Verification items for the finished model (mm, model axes). Coordinates: 2 decimals unless noted, no trailing zeros. Write each loop counter-clockwise with the first axis right and the second up, starting at its lowest first coordinate (ties: lowest second). Pieces come first, ordered by that corner, then holes. Notation, with made-up numbers: (-5, 44.5) -> (43, 44.5) arc R23 ccw to (43, 62.5) -> close; hole circle Ø5 at (69.5, 23). An arc over 180 degrees is marked (long way). Write item = value, one per line. Start each with the question number.
(1) Mould release check, pull along Z, two halves, no side actions. Record for faces 1 (the face through (-44, -154, 26)), 2 (the face through (15.02, -2.15, 47.69)), 3 (the face through (2.64, -2.15, -59.94)): released by +Z, released by -Z, zero draft, split by the parting line, or undercut.
(2) Gauge pin test, flat ends, axial feed: pin 1 Ø3 at (x, z) = (-55, 0) entering from +Y; pin 2 Ø4 at (y, z) = (-120.5, -41) entering from +X; pin 3 Ø3 at (x, y) = (-23, -37) entering from +Z. Record the tip position at first contact, or that the pin passes through.
(3) Section check A-A (y = 126.5). Record the cut outline in (x, z), plus the area to 3 significant figures.
(4) Material ranges on probe 1 along X at (y, z) = (145, 0); probe 2 along X at (y, z) = (125.5, 2); probe 3 along X at (y, z) = (122, -8.5), recorded low to high. Write a range as [from, to].
```python
from build123d import *

# Parameters (mm, degrees)
BOSS_EXTRUDE1_DEPTH              = 154
BOSS_EXTRUDE1_DEPTH_BACK         = 154
SKETCH1_R                        = 60
SKETCH1_R_2                      = 50
TAP_DRILL_FOR_M6_TAP1_AT_2_COUNT = 2
TAP_DRILL_FOR_M6_TAP1_AT_2_PITCH = 42.09517756
TAP_DRILL_FOR_M6_TAP1_AT_3_COUNT = 2
TAP_DRILL_FOR_M6_TAP1_AT_3_PITCH = 77.781745931
TAP_DRILL_FOR_M6_TAP1_AT_4_COUNT = 2
TAP_DRILL_FOR_M6_TAP1_AT_4_PITCH = 101.626748576
TAP_DRILL_FOR_M6_TAP1_AT_5_COUNT = 2
TAP_DRILL_FOR_M6_TAP1_AT_5_PITCH = 110
TAP_DRILL_FOR_M6_TAP1_AT_6_COUNT = 2
TAP_DRILL_FOR_M6_TAP1_AT_6_PITCH = 101.626748576
TAP_DRILL_FOR_M6_TAP1_AT_7_COUNT = 2
TAP_DRILL_FOR_M6_TAP1_AT_7_PITCH = 77.781745931
TAP_DRILL_FOR_M6_TAP1_AT_8_COUNT = 2
TAP_DRILL_FOR_M6_TAP1_AT_8_PITCH = 42.09517756
CHAMFER1_SIZE                    = 0.6


with BuildPart() as part:
    # Sketch1 → Boss-Extrude1 (new, two sides: drawn at the far end of the back side and taken through both)
    with BuildSketch(Plane(origin=(0, 0, 0), x_dir=(1, 0, 0), z_dir=(0, 1, 0)).offset(-BOSS_EXTRUDE1_DEPTH_BACK)):
        with Locations(Location((0, 0, 0), (0, 0, 270))):
            Circle(SKETCH1_R)
        with Locations(Location((0, 0, 0), (0, 0, 270))):
            Circle(SKETCH1_R_2, mode=Mode.SUBTRACT)
    extrude(amount=BOSS_EXTRUDE1_DEPTH + BOSS_EXTRUDE1_DEPTH_BACK)

    # Sketch3 → Tap Drill for M6 Tap1 (revolve, cut)
    with BuildSketch(Plane(origin=(-38.890872965, 154, -38.890872965), x_dir=(0, 0, 1), z_dir=(1, 0, 0))):
        Polygon((0, 0), (0, 16.502151548), (2.5, 15), (2.5, 0), align=None)
    tap_drill_for_m6_tap1 = revolve(axis=Axis((-38.890872965, 160.35, -38.890872965), (0, -1, 0)), mode=Mode.SUBTRACT)

    # Tap Drill for M6 Tap1 at 2: Tap Drill for M6 Tap1 ×2
    with Locations(*[Vector(0.92387953251135, 0, -0.3826834323649371) * (i * TAP_DRILL_FOR_M6_TAP1_AT_2_PITCH) for i in range(1, TAP_DRILL_FOR_M6_TAP1_AT_2_COUNT)]):
        add(tap_drill_for_m6_tap1, mode=Mode.SUBTRACT)

    # Tap Drill for M6 Tap1 at 3: Tap Drill for M6 Tap1 ×2
    with Locations(*[(i * TAP_DRILL_FOR_M6_TAP1_AT_3_PITCH, 0, 0) for i in range(1, TAP_DRILL_FOR_M6_TAP1_AT_3_COUNT)]):
        add(tap_drill_for_m6_tap1, mode=Mode.SUBTRACT)

    # Tap Drill for M6 Tap1 at 4: Tap Drill for M6 Tap1 ×2
    with Locations(*[Vector(0.9238795325112054, 0, 0.3826834323652862) * (i * TAP_DRILL_FOR_M6_TAP1_AT_4_PITCH) for i in range(1, TAP_DRILL_FOR_M6_TAP1_AT_4_COUNT)]):
        add(tap_drill_for_m6_tap1, mode=Mode.SUBTRACT)

    # Tap Drill for M6 Tap1 at 5: Tap Drill for M6 Tap1 ×2
    with Locations(*[Vector(0.7071067811863805, 0, 0.7071067811867146) * (i * TAP_DRILL_FOR_M6_TAP1_AT_5_PITCH) for i in range(1, TAP_DRILL_FOR_M6_TAP1_AT_5_COUNT)]):
        add(tap_drill_for_m6_tap1, mode=Mode.SUBTRACT)

    # Tap Drill for M6 Tap1 at 6: Tap Drill for M6 Tap1 ×2
    with Locations(*[Vector(0.38268343236484964, 0, 0.9238795325113862) * (i * TAP_DRILL_FOR_M6_TAP1_AT_6_PITCH) for i in range(1, TAP_DRILL_FOR_M6_TAP1_AT_6_COUNT)]):
        add(tap_drill_for_m6_tap1, mode=Mode.SUBTRACT)

    # Tap Drill for M6 Tap1 at 7: Tap Drill for M6 Tap1 ×2
    with Locations(*[(0, 0, i * TAP_DRILL_FOR_M6_TAP1_AT_7_PITCH) for i in range(1, TAP_DRILL_FOR_M6_TAP1_AT_7_COUNT)]):
        add(tap_drill_for_m6_tap1, mode=Mode.SUBTRACT)

    # Tap Drill for M6 Tap1 at 8: Tap Drill for M6 Tap1 ×2
    with Locations(*[Vector(-0.38268343236537383, 0, 0.9238795325111692) * (i * TAP_DRILL_FOR_M6_TAP1_AT_8_PITCH) for i in range(1, TAP_DRILL_FOR_M6_TAP1_AT_8_COUNT)]):
        add(tap_drill_for_m6_tap1, mode=Mode.SUBTRACT)

    # Mirror1: Tap Drill for M6 Tap1 across plane
    add(tap_drill_for_m6_tap1.mirror(Plane.ZX), mode=Mode.SUBTRACT)

    # Mirror1 copy 1 sketch → Mirror1 copy 1 (revolve, cut)
    with BuildSketch(Plane(origin=(0, -154, -55), x_dir=(0, 0, 1), z_dir=(1, 0, 0))):
        Polygon((0, 0), (0, -16.502151548), (2.5, -15), (2.5, 0), align=None)
    revolve(axis=Axis((0, -160.35, -55), (0, -1, 0)), mode=Mode.SUBTRACT)

    # Mirror1 copy 2 sketch → Mirror1 copy 2 (revolve, cut)
    with BuildSketch(Plane(origin=(38.890872965, -154, -38.890872965), x_dir=(0, 0, 1), z_dir=(1, 0, 0))):
        Polygon((0, 0), (0, -16.502151548), (2.5, -15), (2.5, 0), align=None)
    revolve(axis=Axis((38.890872965, -160.35, -38.890872965), (0, -1, 0)), mode=Mode.SUBTRACT)

    # Mirror1 copy 3 sketch → Mirror1 copy 3 (revolve, cut)
    with BuildSketch(Plane(origin=(55, -154, 0), x_dir=(0, 0, 1), z_dir=(1, 0, 0))):
        Polygon((0, 0), (0, -16.502151548), (2.5, -15), (2.5, 0), align=None)
    revolve(axis=Axis((55, -160.35, 0), (0, -1, 0)), mode=Mode.SUBTRACT)

    # Mirror1 copy 4 sketch → Mirror1 copy 4 (revolve, cut)
    with BuildSketch(Plane(origin=(38.890872965, -154, 38.890872965), x_dir=(0, 0, 1), z_dir=(1, 0, 0))):
        Polygon((0, 0), (0, -16.502151548), (2.5, -15), (2.5, 0), align=None)
    revolve(axis=Axis((38.890872965, -160.35, 38.890872965), (0, -1, 0)), mode=Mode.SUBTRACT)

    # Mirror1 copy 5 sketch → Mirror1 copy 5 (revolve, cut)
    with BuildSketch(Plane(origin=(0, -154, 55), x_dir=(0, 0, 1), z_dir=(1, 0, 0))):
        Polygon((0, 0), (0, -16.502151548), (2.5, -15), (2.5, 0), align=None)
    revolve(axis=Axis((0, -160.35, 55), (0, -1, 0)), mode=Mode.SUBTRACT)

    # Mirror1 copy 6 sketch → Mirror1 copy 6 (revolve, cut)
    with BuildSketch(Plane(origin=(-38.890872965, -154, 38.890872965), x_dir=(0, 0, 1), z_dir=(1, 0, 0))):
        Polygon((0, 0), (0, -16.502151548), (2.5, -15), (2.5, 0), align=None)
    revolve(axis=Axis((-38.890872965, -160.35, 38.890872965), (0, -1, 0)), mode=Mode.SUBTRACT)

    # Mirror1 copy 7 sketch → Mirror1 copy 7 (revolve, cut)
    with BuildSketch(Plane(origin=(-55, -154, 0), x_dir=(0, 0, 1), z_dir=(1, 0, 0))):
        Polygon((0, 0), (0, -16.502151548), (2.5, -15), (2.5, 0), align=None)
    revolve(axis=Axis((-55, -160.35, 0), (0, -1, 0)), mode=Mode.SUBTRACT)

    # Chamfer1
    chamfer1_edges = [part.edges().sort_by_distance(p)[0] for p in [
        (0, 154, -60),
        (0, 154, -50),
        (0, -154, -60),
        (0, -154, -50),
    ]]
    chamfer(chamfer1_edges, length=CHAMFER1_SIZE)


solid = part.part
```
Response:
q1.face_1 = zero draft
q1.face_2 = undercut
q1.face_3 = split by the parting line
q2.pin_1 = 138.4
q2.pin_2 = 45.6
q2.pin_3 = 56.02
q3.outline = circle Ø120 at (0, 0); hole circle Ø100 at (0, 0)
q3.area = 3,460 mm2
q4.probe_1 = [-60, -57.5], [-52.5, -50], [50, 52.5], [57.5, 60]
q4.probe_2 = [-59.97, -49.96], [49.96, 59.97]
q4.probe_3 = [-59.39, -49.27], [49.27, 59.39]
